The listing builds one solid part. Answer for the finished solid, in the listing's coordinates (mm). Face numbers are marked on the shaded views. A direction names the side the tool comes from. Round coordinates to 2 decimals unless told otherwise and drop trailing zeros. Write each loop counter-clockwise with the first axis right and the second up, starting at its lowest first coordinate (ties: lowest second). Pieces come first, ordered by that corner, then holes. Notation, with made-up numbers: (76, -30.5) - (103, -30.5) arc R36 ccw to (103, 7.5) - close; hole circle Ø9 at (52.25, 54.5). An arc over 180 degrees is marked (long way). Use a Markdown table: item, result. Add a question column.
1) A tool of negligible diameter and unlimited length cuts with its end or side. For the marked faces 1, 2, 3, 4 and 5, from which of +Z, -Z, +X, -X, +Y, -Y can it reach the whole face along a straight path? Write none if from no direction.
2) Each of these flat-tipped pins is pushed along its axis until it touches: P1, Ø3, axis at y = 5.5, z = -0.5, coming from the +X side; P2, Ø3, axis at y = 3.5, z = -4, coming from the +X side; P3, Ø1.6, axis at x = -10.5, z = -5.5, coming from the -Y side. Where does it stop, or does it pass through?
3) A cutting plane is placed at B-B (z = -8). Give the vertices of the cut face in (x, y).
4) A cutting plane is placed at D-D (z = -10). Give the vertices of the cut face in (x, y).
5) A cutting plane is placed at A-A (y = 0). Give the vertices of the cut face in (x, z).
6) Find the intervals of material crossed by probe 1 along Y at (x, z) = (0, -9); probe 2 along X at (y, z) = (3.5, -4); probe 3 along X at (y, z) = (-1.75, -3), in increasing order. Write a range as from..to.
```python
from build123d import *

# Parameters (mm, degrees)
CUT_EXTRUDE1_DEPTH       = 10
BOSS_EXTRUDE1_DEPTH      = 9
BOSS_EXTRUDE1_DEPTH_BACK = 1
SKETCH4_W                = 3.1346611
SKETCH4_H                = 1


with BuildPart() as part:
    # Sketch2 → Revolve1 (revolve)
    with BuildSketch(Plane(origin=(0, 0, 0), x_dir=(1, 0, 0), z_dir=(0, 1, 0)), mode=Mode.PRIVATE) as revolve1_sk:
        with BuildLine():
            Line((4, 11), (4, 2))
            ThreePointArc((4, 2), (4.878679656, -0.121320344), (7, -1))
            Line((7, -1), (12.5, -1))
            Line((12.5, -1), (12.5, 0))
            Line((12.5, 0), (7, 0))
            ThreePointArc((7, 0), (5.585786438, 0.585786438), (5, 2))
            Line((5, 2), (5, 11))
            Line((5, 11), (4, 11))
        make_face()
    revolve(revolve1_sk.sketch.rotate(Axis((0, 0, -90.408402744), (0, 0, 1)), 180), axis=Axis((0, 0, -90.408402744), (0, 0, 1)))

    # Sketch3 → Cut-Extrude1 (cut)
    with BuildSketch(Plane(origin=(0, 0, 0), x_dir=(-1, 0, 0), z_dir=(0, 0, -1))):
        with BuildLine():
            Line((9, 8.674675786), (9, 3))
            Line((9, 3), (12.1346611, 3))
            ThreePointArc((12.1346611, 3), (10.941616026, 6.044091225), (9, 8.674675786))
        make_face()
        with BuildLine():
            Line((8.674675786, -9), (3, -9))
            Line((3, -9), (3, -12.1346611))
            ThreePointArc((3, -12.1346611), (6.044091225, -10.941616026), (8.674675786, -9))
        make_face()
        with BuildLine():
            Line((-9, -8.674675786), (-9, -3))
            Line((-9, -3), (-12.1346611, -3))
            ThreePointArc((-12.1346611, -3), (-10.941616026, -6.044091225), (-9, -8.674675786))
        make_face()
        with BuildLine():
            Line((-8.674675786, 9), (-3, 9))
            Line((-3, 9), (-3, 12.1346611))
            ThreePointArc((-3, 12.1346611), (-6.044091225, 10.941616026), (-8.674675786, 9))
        make_face()
    extrude(amount=-CUT_EXTRUDE1_DEPTH, mode=Mode.SUBTRACT)

    # Sketch4 → Boss-Extrude1 (add, two sides: drawn at the far end of the back side and taken through both)
    with BuildSketch(Plane(origin=(0, 0, 0), x_dir=(-1, 0, 0), z_dir=(0, 0, -1)).offset(-BOSS_EXTRUDE1_DEPTH_BACK)):
        with Locations((10.56733055, 3.5)):
            Rectangle(SKETCH4_W, SKETCH4_H)
    extrude(amount=BOSS_EXTRUDE1_DEPTH + BOSS_EXTRUDE1_DEPTH_BACK)


solid = part.part
```
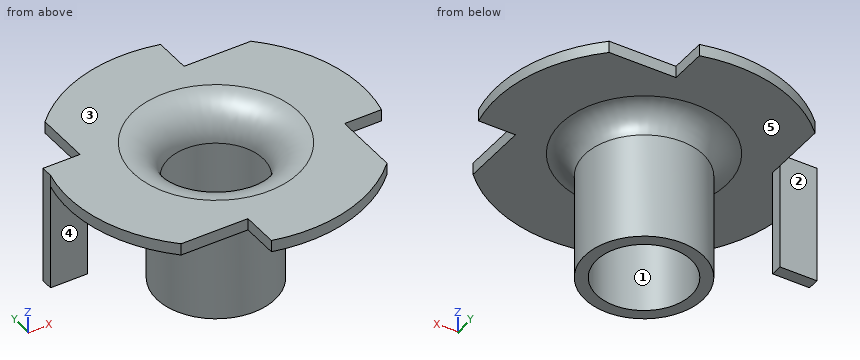
Entries:
| question | item | result |
|---|---|---|
| 1 | face 1 | +Z, -Z |
| 1 | face 2 | +Z, -Z, -X, +Y |
| 1 | face 3 | +Z, +X, -X, +Y, -Y |
| 1 | face 4 | -Z, -X, -Y |
| 1 | face 5 | -Z |
| 2 | P1 | stops at x = 11.81 |
| 2 | P2 | stops at x = 4.58 |
| 2 | P3 | stops at y = 3 |
| 3 | outline | (-12.13, 3) - (-9, 3) - (-9, 4) - (-12.13, 4) - close; circle Ø10 at (0, 0); hole circle Ø8 at (0, 0) |
| 4 | outline | circle Ø10 at (0, 0); hole circle Ø8 at (0, 0) |
| 5 | outline | (-12.5, 0) - (-7, 0) arc R2 cw to (-5, -2) - (-5, -11) - (-4, -11) - (-4, -2) arc R3 ccw to (-7, 1) - (-12.5, 1) - close; (4, -11) - (5, -11) - (5, -2) arc R2 cw to (7, 0) - (12.5, 0) - (12.5, 1) - (7, 1) arc R3 ccw to (4, -2) - close |
| 6 | probe 1 | y = -5..-4, 4..5 |
| 6 | probe 2 | x = -12.13..-9, -3.57..-1.94, 1.94..3.57 |
| 6 | probe 3 | x = -4.68..-3.6, 3.6..4.68 |
